from build123d import *

# Parameters (mm, degrees)
F1_DEPTH = 4
F2_W     = 47.247536
F2_H     = 16.5
F3_DEPTH = 2


with BuildPart() as f1:
    # F0 (on Top) → F1 (new body)
    with BuildSketch(Plane.XY):
        with BuildLine():
            ThreePointArc((0, 27.313505), (-9.686066, 22.852633), (-12.592393, 12.592393))
            ThreePointArc((-12.592393, 12.592393), (-27.313505, 0), (-12.592393, -12.592393))
            ThreePointArc((-12.592393, -12.592393), (0, -27.313505), (12.592393, -12.592393))
            ThreePointArc((12.592393, -12.592393), (27.313505, 0), (12.592393, 12.592393))
            ThreePointArc((12.592393, 12.592393), (9.686066, 22.852633), (0, 27.313505))
        make_face()
        with BuildLine():
            ThreePointArc((0, 18.440354), (-2.5, 20.940354), (0, 23.440354))
            ThreePointArc((0, 23.440354), (1.767767, 22.708121), (2.5, 20.940354))
            ThreePointArc((2.5, 20.940354), (1.767767, 19.172587), (0, 18.440354))
        make_face(mode=Mode.SUBTRACT)
    extrude(amount=F1_DEPTH)

    # F2 (on face) → F3 (cut)
    with BuildSketch(Plane.XY.offset(4)):
        Rectangle(F2_W, F2_H)
    extrude(amount=-F3_DEPTH, mode=Mode.SUBTRACT)


solid = f1.part
For this review, take the finished solid that the model builds, in its own axes (mm). A direction names the side the tool comes from. Round coordinates to 2 decimals unless told otherwise and drop trailing zeros. Loops run counter-clockwise (first coordinate to the right, second up) from the corner with the lowest first, then second, coordinate; pieces in that order, holes last. Notation, with made-up numbers: (39, -29.75) - (84, -29.75) arc R22 ccw to (84, -23.75) - close; hole circle Ø1 at (34.25, -31.75). An arc over 180 degrees is marked (long way). One line per item, written item: value. Start each with the question number.
Item 1: For faces 3 (the flat face through (0, -12, 4)), 4 (the flat face through (0, -8.25, 3)), list the 3-axis set-ups (+Z, -Z, +X, -X, +Y, -Y) from which the entire face can be reached by the end or side of a thin tool; tool diameter is ignored.
Item 2: Clearance check with flat-ended pins moving along their axes: pin 1 Ø1 at (y, z) = (-6, 3) entering from -X; pin 2 Ø2 at (y, z) = (-0.5, 3) entering from -X; pin 3 Ø1 at (y, z) = (2.5, 2.5) entering from +X; pin 4 Ø5 at (x, y) = (-10, -0.5) entering from +Z. State where each tip first meets the part, or that it passes through.
Item 3: Take a section at C-C (x = -23). Give the boundary of the cut face in (y, z), plus the area to 3 significant figures.
Item 4: For L1, parallel to Z at x = 19, y = 5; L2, parallel to Y at x = 1.5, z = 3.65; L3, parallel to X at y = 7, z = 3.4, list the stretches that pass through material, from the lowest coordinate up.
Item 5: Take a section at B-B (y = 0). Give the boundary of the cut face in (x, z).
Item 6: The part is to be moulded in two halves that separate along X. For faces 1 (the flat face through (23.624, 0, 3)), 2 (the flat face through (0, 0, 0)), say which applies: +X half, -X half, draft (parallel to the pull), parting line (faces both ways), or undercut.
Item 7: Take a section at D-D (x = 1.5). Give the boundary of the cut face in (y, z), plus the area to 3 significant figures.
Item 8: Take a section at A-A (z = 1). Give the boundary of the cut face in (x, y).
Answer below:
1. face 3: +Z, +X, -X, +Y, -Y
1. face 4: +Z
2. pin 1: stops at x = -26.07
2. pin 2: stops at x = -27.31
2. pin 3: stops at x = 27.16
2. pin 4: stops at z = 2
3. outline: (-9.56, 0) - (9.56, 0) - (9.56, 4) - (8.25, 4) - (8.25, 2) - (-8.25, 2) - (-8.25, 4) - (-9.56, 4) - close
3. area: 43.5 mm2
4. L1: z = 0 to 2
4. L2: y = -27.22 to -8.25, 8.25 to 18.94, 22.94 to 27.22
4. L3: x = -25.22 to -23.62, 23.62 to 25.22
5. outline: (-27.31, 0) - (27.31, 0) - (27.31, 4) - (23.62, 4) - (23.62, 2) - (-23.62, 2) - (-23.62, 4) - (-27.31, 4) - close
6. face 1: undercut
6. face 2: draft
7. outline: (-27.22, 0) - (18.94, 0) - (18.94, 4) - (8.25, 4) - (8.25, 2) - (-8.25, 2) - (-8.25, 4) - (-27.22, 4) - close; (22.94, 0) - (27.22, 0) - (27.22, 4) - (22.94, 4) - close
7. area: 169 mm2
8. outline: (-12.59, -12.59) arc R12.75 ccw (long way) to (12.59, -12.59) arc R12.75 ccw (long way) to (12.59, 12.59) arc R12.75 ccw (long way) to (-12.59, 12.59) arc R12.75 ccw (long way) to start; hole circle Ø5 at (0, 20.94)
